The model under review builds one solid part; all positions refer to its coordinate system, in mm. A direction names the side the tool comes from. Round coordinates to 2 decimals unless told otherwise and drop trailing zeros. Write each loop counter-clockwise with the first axis right and the second up, starting at its lowest first coordinate (ties: lowest second). Pieces come first, ordered by that corner, then holes. Notation, with made-up numbers: (0, 48) - (46, 48) arc R12 cw to (46, 64) - close; hole circle Ø6 at (26.5, -28). An arc over 180 degrees is marked (long way). Use one line per item in the form item = value.
from build123d import *

# Parameters (mm, degrees)
SKETCH1_R                = 7.5
BOSS_EXTRUDE1_DEPTH      = 1
BOSS_EXTRUDE2_DEPTH      = 1
BOSS_EXTRUDE2_DEPTH_BACK = 1
SKETCH5_R                = 1.5
BOSS_EXTRUDE3_DEPTH      = 7
CHAMFER1_SIZE            = 0.2


with BuildPart() as part:
    # Sketch1 → Boss-Extrude1 (new body)
    with BuildSketch(Plane(origin=(0, 0, 0), x_dir=(1, 0, 0), z_dir=(0, 1, 0))):
        with Locations(Location((0, 0, 0), (0, 0, 270))):
            Circle(SKETCH1_R)
    extrude(amount=BOSS_EXTRUDE1_DEPTH)

    # Sketch3 → Revolve1 (revolve)
    with BuildSketch(Plane.XY):
        with BuildLine():
            Line((0, 1), (0, 3))
            add(Edge.make_bspline(
                [(7.5, 1), (4.015025373, 2.967534518), (0, 3)],
                knots=[0, 0, 0, 1, 1, 1], degree=2))
            Line((7.5, 1), (0, 1))
        make_face()
    revolve(axis=Axis((0, 1, 0), (0, 1, 0)))

    # Sketch4 → Boss-Extrude2 (add, two sides: drawn at the far end of the back side and taken through both)
    with BuildSketch(Plane(origin=(0, 0, 0), x_dir=(0, 0, -1), z_dir=(1, 0, 0)).offset(-BOSS_EXTRUDE2_DEPTH_BACK)):
        Polygon((-7.5, 1), (-3.499989483, 1), (3.500010517, 1), (7.5, 1), (3.500010517, 5), (-3.499989483, 5), align=None)
    extrude(amount=BOSS_EXTRUDE2_DEPTH + BOSS_EXTRUDE2_DEPTH_BACK)

    # Sketch5 → Boss-Extrude3 (add)
    with BuildSketch(Plane.XZ):
        with Locations(Location((0, 0, 0), (0, 0, 270))):
            Circle(SKETCH5_R)
    extrude(amount=BOSS_EXTRUDE3_DEPTH)

    # Chamfer1
    chamfer1_edges = [part.edges().sort_by_distance(p)[0] for p in [
        (0, -7, 1.5),
    ]]
    chamfer(chamfer1_edges, length=CHAMFER1_SIZE)


solid = part.part
(1) Add section A-A on y = 0.25. Write out the cut boundary in (x, z).
Geometry results:
outline = circle Ø15 at (0, 0)
(2) Add section B-B on y = -3. Write out the cut boundary in (x, z), then the cut area to 3 significant figures.
Geometry results:
outline = circle Ø3 at (0, 0)
area = 7.07 mm2
(3) Insertion check: P1, Ø1, axis at x = 5.5, y = 0.5, coming from the -Z side; P2, Ø5, axis at x = -5.5, z = -2, coming from the -Y side; P3, Ø4.5, axis at y = 2, z = 2, coming from the -X side; P4, Ø3, axis at y = -0.5, z = -5.5, coming from the -X side. Each pin has a flat end and moves straight along its axis. Give the tip position at first contact, or say it passes through.
Geometry results:
P1 = -5.59
P2 = 0
P3 = -7.5
P4 = -6.29
(4) To check wall thickness, follow L1, parallel to X at y = 3.25, z = 2.5; L2, parallel to Y at x = 6, z = 3.5; L3, parallel to Y at x = 3, z = 5.25. State the ranges of each line that lie inside material, in increasing order.
Geometry results:
L1 = -1 to 1
L2 = 0 to 1.3
L3 = 0 to 1.73
(5) Machinability: for faces 1 (the cylindrical face through (0.45, -3.35, -1.43)), 2 (the flat face through (0, -7, 0)), which of the approach directions +Z, -Z, +X, -X, +Y, -Y give a long, thin tool a straight path to every point of the face, cutting with its end or side? Answer none if there is none.
Geometry results:
face_1 = -Y
face_2 = +Z, -Z, +X, -X, -Y
